```python
from build123d import *

# Parameters (mm, degrees)
SKETCH1_R           = 16.5
BOSS_EXTRUDE1_DEPTH = 22.5
SKETCH2_R           = 18.5
BOSS_EXTRUDE2_DEPTH = 18.25
SKETCH7_R           = 1.5
CUT_EXTRUDE2_DEPTH  = 6


with BuildPart() as part:
    # Sketch1 → Boss-Extrude1 (new body)
    with BuildSketch(Plane(origin=(0, 0, 0), x_dir=(1, 0, 0), z_dir=(0, 1, 0))):
        with Locations(Location((0, 0, 0), (0, 0, 90))):
            Circle(SKETCH1_R)
    extrude(amount=BOSS_EXTRUDE1_DEPTH)

    # Sketch2 → Boss-Extrude2 (add)
    with BuildSketch(Plane(origin=(0, 22.5, 0), x_dir=(1, 0, 0), z_dir=(0, 1, 0))):
        with Locations(Location((0, 0, 0), (0, 0, 270))):
            Circle(SKETCH2_R)
    extrude(amount=BOSS_EXTRUDE2_DEPTH)

    # Sketch7 → Cut-Extrude2 (cut)
    with BuildSketch(Plane(origin=(0, 40.75, 0), x_dir=(1, 0, 0), z_dir=(0, 1, 0))):
        with Locations(Location((15.5, 0, 0), (0, 0, 270))):
            Circle(SKETCH7_R)
        with Locations(Location((7.75, 13.423393759, 0), (0, 0, 270))):
            Circle(SKETCH7_R)
        with Locations(Location((-15.5, 0, 0), (0, 0, 90))):
            Circle(SKETCH7_R)
        with Locations(Location((-7.75, 13.423393759, 0), (0, 0, 90))):
            Circle(SKETCH7_R)
        with Locations(Location((7.75, -13.423393759, 0), (0, 0, 90))):
            Circle(SKETCH7_R)
        with Locations(Location((-7.75, -13.423393759, 0), (0, 0, 270))):
            Circle(SKETCH7_R)
    extrude(amount=-CUT_EXTRUDE2_DEPTH, mode=Mode.SUBTRACT)


solid = part.part
```
Can you work these out from the model? Positions are in its coordinate system, mm. A direction names the side the tool comes from. Round coordinates to 2 decimals unless told otherwise and drop trailing zeros. Loops run counter-clockwise (first coordinate to the right, second up) from the corner with the lowest first, then second, coordinate; pieces in that order, holes last. Notation, with made-up numbers: M -11,41.25 L 27,41.25 A17 cw 27,53.25 Z; hole C 49.5,61.5 d9. An arc over 180 degrees is marked long. Answer in a Markdown table with one row per item.
1. If we section it at D-D, the plane x = -7.75: Please give me the cut outline in (y, z), plus the area to 3 significant figures.
Established:
| item | result |
|---|---|
| outline | M 0,-14.57 L 22.5,-14.57 L 22.5,-16.8 L 40.75,-16.8 L 40.75,-14.92 L 34.75,-14.92 L 34.75,-11.92 L 40.75,-11.92 L 40.75,11.92 L 34.75,11.92 L 34.75,14.92 L 40.75,14.92 L 40.75,16.8 L 22.5,16.8 L 22.5,14.57 L 0,14.57 Z |
| area | 1,230 mm² |
2. Thinking about a two-plate mould opening in Z: for faces 1 (the face through (-7.086, 31.497, 17.089)), 2 (the face through (0, 0, 0)), 3 (the face through (8, 34.75, 13)), which applies, pulls with the +Z half, pulls with the -Z half, needs draft (parallel to the pull), parting line crosses it, or undercut?
Established:
| item | result |
|---|---|
| face 1 | parting line crosses it |
| face 2 | needs draft |
| face 3 | undercut |
3. If we section it at A-A, the plane x = 0: Please give me the cut outline in (y, z), plus the area to 3 significant figures.
Established:
| item | result |
|---|---|
| outline | M 0,-16.5 L 22.5,-16.5 L 22.5,-18.5 L 40.75,-18.5 L 40.75,18.5 L 22.5,18.5 L 22.5,16.5 L 0,16.5 Z |
| area | 1,420 mm² |
4. On a 3-axis mill with a long thin cutter (end or side, diameter ignored), from which of +Z, -Z, +X, -X, +Y, -Y can I reach the whole of each face in a straight line? I mean faces 4 (the face through (-6.84, 37.79, -12.23)), 5 (the face through (0, 40.75, 0)), 6 (the face through (16.108, 11.092, 3.577)). Say none if no direction works.
Established:
| item | result |
|---|---|
| face 4 | +Y |
| face 5 | +Z, -Z, +X, -X, +Y |
| face 6 | -Y |
5. If we section it at C-C, the plane y = 3: Please give me the cut outline in (x, z).
Established:
| item | result |
|---|---|
| outline | C 0,0 d33 |
6. Please list where these lines run through material, in increasing order: line 1 (X direction, y = 36.5, z = 0); line 2 (Z direction, x = 7, y = 39); line 3 (Y direction, x = 16.5, z = 3.5). Write a range as from..to.
Established:
| item | result |
|---|---|
| line 1 | -18.5..-17, -14..14, 17..18.5 |
| line 2 | -17.12..-14.72, -12.12..12.12, 14.72..17.12 |
| line 3 | 22.5..40.75 |
7. If we section it at B-B, the plane z = 9: Please give me the cut outline in (x, y), plus the area to 3 significant figures.
Established:
| item | result |
|---|---|
| outline | M -16.16,22.5 L -13.83,22.5 L -13.83,0 L 13.83,0 L 13.83,22.5 L 16.16,22.5 L 16.16,40.75 L -16.16,40.75 Z |
| area | 1,210 mm² |
8. I'm going to push flat-ended pins straight in: pin 1 Ø4 at (y, z) = (26.5, 8.5) entering from -X; pin 2 Ø1 at (x, y) = (-8.5, 14.5) entering from -Z; pin 3 Ø10 at (y, z) = (35, -10) entering from +X. Where does each tip first touch, or does it pass through?
Established:
| item | result |
|---|---|
| pin 1 | x = -17.32 |
| pin 2 | z = -14.43 |
| pin 3 | x = 17.81 |
